Read the model definition and answer for the solid it produces. Units are mm, in the model's axes. Face numbers are marked on the shaded views. A direction names the side the tool comes from. Give positions to 0.01 mm unless a question says otherwise; leave off trailing zeros. Loops run counter-clockwise (first coordinate to the right, second up) from the corner with the lowest first, then second, coordinate; pieces in that order, holes last. Notation, with made-up numbers: (74.5, 27.5) - (81.5, 27.5) arc R28 ccw to (81.5, 54.5) - close; hole circle Ø11 at (74.5, 65). An arc over 180 degrees is marked (long way). Put each result on its own line as item: value. Start each with the question number.
1. For a pull along Z with two mould halves and no side action, classify the marked faces 4, 5, 6 and 7 as released by +Z, released by -Z, zero draft, split by the parting line, or undercut.
2. A cutting plane is placed at A-A, the plane z = -41. Determine the outline of the cut face in (x, y), plus the area to 3 significant figures.
3. A cutting plane is placed at D-D, the plane z = -101. Determine the outline of the cut face in (x, y).
4. A cutting plane is placed at B-B, the plane y = 32.5. Determine the outline of the cut face in (x, z).
5. For the marked faces 1, 2 and 3, determine the directions among +Z, -Z, +X, -X, +Y, -Y from which every point of the face is accessible in a straight line to the end or side of a thin tool.
6. A cutting plane is placed at C-C, the plane x = -49. Determine the outline of the cut face in (y, z), plus the area to 3 significant figures.
7. Consider L1, parallel to X at y = 41.55, z = 5; L2, parallel to Z at x = -20, y = 16; L3, parallel to Z at x = -99, y = 40.1. Determine where each line is inside the solid, lowest interval first. Write a range as from..to.
8. Given pin 1 Ø5 at (x, z) = (-97, -159) entering from -Y; pin 2 Ø2 at (x, y) = (-117.5, 9) entering from -Z; pin 3 Ø10 at (x, y) = (-61.5, 32) entering from +Z, each flat-ended and moving along its own axis, determine where each tip first touches the part or whether it passes through.
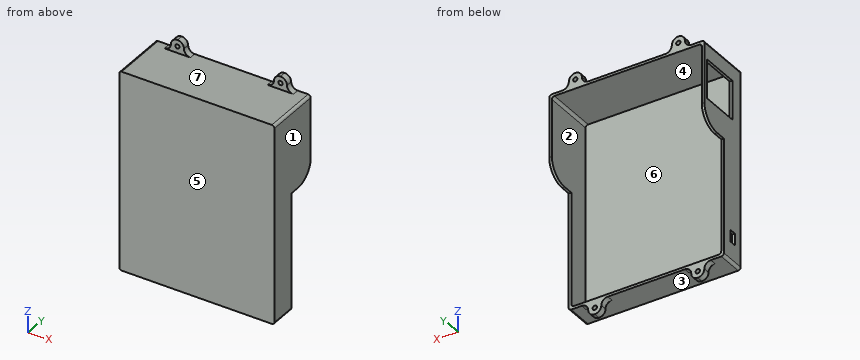
Autodesk Inventor part; units mm, degrees
ref_plane "YZ Plane" through (0, 0, 0) normal (1, 0, 0) x (0, 1, 0)
ref_plane "XZ Plane" through (0, 0, 0) normal (0, 1, 0) x (-1, 0, 0)
ref_plane "XY Plane" through (0, 0, 0) normal (0, 0, 1) x (1, 0, 0)
sketch "Sketch2" plane through (0, 0, 0) normal (0, 1, 0) x (-1, 0, 0)
  line L0 (0, 0) -> (119, 0)
  line L1 (119, 0) -> (119, -153)
  line L2 (119, -153) -> (0, -153)
  line L3 (0, -153) -> (0, 0)
  dimension "d0" = 119
  dimension "d1" = 153
extrude "Extrusion1" add sketch "Sketch2" along normal blind 3
sketch "Sketch7" plane through (0, 3, 0) normal (0, 1, 0) x (1, 0, 0)
  line L0 (-117, 2) -> (-2, 2)
  line L1 (-2, 2) -> (-2, 151)
  line L2 (-2, 151) -> (-117, 151)
  line L3 (-117, 151) -> (-117, 2)
  line L4 (-119, 153) -> (-119, 0)
  line L5 (-119, 0) -> (0, 0)
  line L6 (0, 153) -> (-119, 153)
  line L7 (-119, 0) -> (0, 0)
  line L8 (0, 0) -> (0, 153)
  line L9 (0, 153) -> (-119, 153)
  line L10 (-119, 153) -> (-119, 0)
  dimension "d27" = 115
  dimension "d28" = 149
  dimension "d29" = 2
  dimension "d30" = 2
extrude "Extrusion5" add sketch "Sketch7" along normal blind 17
sketch "Sketch8" plane through (0, 20, 0) normal (0, 1, 0) x (1, 0, 0)
  line L0 (-119, 0) -> (0, 0)
  line L1 (-119, 0) -> (0, 0)
  line L2 (0, 0) -> (0, 63)
  line L3 (-119, 63) -> (-119, 0)
  line L4 (-117, 2) -> (-117, 151)
  line L5 (-2, 151) -> (-2, 2)
  line L6 (-117, 2) -> (-2, 2)
  line L7 (-2, 2) -> (-2, 63)
  line L8 (-2, 63) -> (-117, 63)
  line L9 (-117, 63) -> (-117, 2)
  line L10 (0, 63) -> (-2, 63)
  line L11 (-117, 63) -> (-119, 63)
  dimension "d33" = 119
  dimension "d34" = 63
extrude "Extrusion6" add sketch "Sketch8" along normal blind 23 contours L3 L11 L4 L6 L5 L10 L2 L0
sketch "Sketch9" plane through (-119, 0, -153) normal (-1, 0, 0) x (0, 0, 1)
  line L0 (15, 12) -> (24, 12)
  line L1 (24, 12) -> (24, 7)
  line L2 (24, 7) -> (15, 7)
  line L3 (15, 7) -> (15, 12)
  line L4 (2, 3) -> (151, 3)
  line L5 (0, 0) -> (0, 20)
  line L6 (2, 3) -> (2, 20)
  line L7 (110, 40) -> (140, 40)
  line L8 (140, 40) -> (140, 10)
  line L9 (140, 10) -> (110, 10)
  line L10 (110, 10) -> (110, 40)
  line L11 (0, 0) -> (153, 0)
  line L12 (90, 20) -> (90, 43)
  dimension "d37" = 9
  dimension "d38" = 5
  dimension "d39" = 4
  dimension "d40" = 15
  dimension "d41" = 13
  dimension "d42" = 30
  dimension "d43" = 30
  dimension "d44" = 10
  dimension "d45" = 20
extrude "Extrusion7" cut sketch "Sketch9" against normal blind 23
fillet "Fillet1" radius 2 8 edges at (-119, 10, -153) (-117, 11.5, -151) (0, 21.5, 0) (0, 10, -153) (-119, 21.5, 0) (-2, 23, -2) (-2, 11.5, -151) (-117, 23, -2)
fillet "Fillet2" radius 15 2 edges at (-118, 43, -63) (-1, 43, -63)
sketch "Sketch10" plane through (-117, 0, 0) normal (0, 0, 1) x (1, 0, 0)
  line L0 (113, 43) -> (2, 43)
  line L1 (13, 43) -> (23, 43)
  line L2 (23, 43) -> (23, 38)
  line L3 (23, 38) -> (13, 38)
  line L4 (13, 38) -> (13, 43)
  line L5 (92, 43) -> (102, 43)
  line L6 (102, 43) -> (102, 38)
  line L7 (102, 38) -> (92, 38)
  line L8 (92, 38) -> (92, 43)
  line L9 (117, 0) -> (117, 43)
  line L10 (-2, 43) -> (-2, 0)
  point P0 (23, 43)
  dimension "d50" = 10
  dimension "d51" = 5
  dimension "d52" = 10
  dimension "d53" = 5
  dimension "d54" = 119
  dimension "d55" = 15
  dimension "d56" = 15
extrude "Extrusion8" add sketch "Sketch10" along normal blind 10
sketch "Sketch11" plane through (-2, 0, -153) normal (0, 0, -1) x (-1, 0, 0)
  line L0 (113, 20) -> (2, 20)
  line L1 (13, 20) -> (23, 20)
  line L2 (23, 20) -> (23, 15)
  line L3 (23, 15) -> (13, 15)
  line L4 (13, 15) -> (13, 20)
  line L5 (92, 20) -> (102, 20)
  line L6 (102, 20) -> (102, 15)
  line L7 (102, 15) -> (92, 15)
  line L8 (92, 15) -> (92, 20)
  line L9 (-2, 20) -> (-2, 0)
  line L10 (117, 0) -> (117, 20)
  dimension "d59" = 10
  dimension "d60" = 5
  dimension "d61" = 10
  dimension "d62" = 5
  dimension "d63" = 15
  dimension "d64" = 15
extrude "Extrusion9" add sketch "Sketch11" along normal blind 10
sketch "Sketch12" plane through (0, 43, 0) normal (0, 1, 0) x (1, 0, 0)
  circle A0 centre (-99, -5) radius 1.65
  line L0 (-94, -10) -> (-104, -10)
  circle A1 centre (-20, -5) radius 1.65
  line L1 (-15, -10) -> (-25, -10)
  line L2 (-104, 0) -> (-104, -10)
  line L3 (-15, 0) -> (-15, -10)
  point P0 (0, 0)
  dimension "d67" = 3.3
  dimension "d68" = 5
  dimension "d69" = 3.3
  dimension "d70" = 5
  dimension "d71" = 5
  dimension "d72" = 5
extrude "Extrusion10" cut sketch "Sketch12" against normal blind 10
sketch "Sketch13" plane through (0, 20, 0) normal (0, 1, 0) x (1, 0, 0)
  circle A0 centre (-99, 158) radius 1.65
  line L0 (-104, 153) -> (-104, 163)
  line L1 (-104, 163) -> (-94, 163)
  circle A1 centre (-20, 158) radius 1.65
  line L2 (-25, 153) -> (-25, 163)
  line L3 (-25, 163) -> (-15, 163)
  point P0 (0, 0)
  point P1 (-25, 158)
  dimension "d75" = 3.3
  dimension "d76" = 5
  dimension "d77" = 5
  dimension "d78" = 3.3
  dimension "d79" = 5
  dimension "d80" = 5
extrude "Extrusion11" cut sketch "Sketch13" against normal blind 10
fillet "Fillet3" radius 5 16 edges at (-15, 17.5, -163) (-25, 17.5, -163) (-15, 17.5, -153) (-94, 17.5, -163) (-94, 17.5, -153) (-25, 17.5, -153) (-104, 17.5, -163) (-104, 17.5, -153) (-104, 40.5, 0) (-104, 40.5, 10) (-94, 40.5, 10) (-94, 40.5, 0) (-25, 40.5, 10) (-15, 40.5, 10) (-15, 40.5, 0) (-25, 40.5, 0)
properties part number "base"
Return value:
1. face 4: undercut
1. face 5: zero draft
1. face 6: undercut
1. face 7: released by +Z
2. outline: (-119, 0) - (0, 0) - (0, 43) - (-2, 43) - (-2, 3) - (-117, 3) - (-117, 10) - (-119, 10) - close; (-119, 40) - (-117, 40) - (-117, 43) - (-119, 43) - close
2. area: 457 mm2
3. outline: (-119, 0) - (0, 0) - (0, 20) - (-2, 20) - (-2, 3) - (-117, 3) - (-117, 20) - (-119, 20) - close
4. outline: (-119, -62.31) - (-117, -62.31) - (-117, -43) - (-119, -43) - close; (-119, -13) - (-117, -13) - (-117, -4) arc R2 cw to (-115, -2) - (-4, -2) arc R2 cw to (-2, -4) - (-2, -62.31) - (0, -62.31) - (0, -2) arc R2 ccw to (-2, 0) - (-117, 0) arc R2 ccw to (-119, -2) - close
5. face 1: +Z, -Z, +X, +Y, -Y
5. face 2: +Y
5. face 3: -Z, -Y
6. outline: (0, -153) - (20, -153) - (20, -151) - (3, -151) - (3, -2) - (43, -2) - (43, 0) - (0, 0) - close
6. area: 573 mm2
7. L1: x = -104..-100.65, -97.35..-94, -25..-21.65, -18.35..-15
7. L2: z = -163..-159.65, -156.35..-151, -2..0
7. L3: z = -2..3.35, 6.65..10
8. pin 1: stops at y = 15
8. pin 2: stops at z = -153
8. pin 3: stops at z = 0
